Part model, mm, in its own coordinate system. A direction names the side the tool comes from. Give positions to 0.01 mm unless a question says otherwise; leave off trailing zeros. Loops run counter-clockwise (first coordinate to the right, second up) from the corner with the lowest first, then second, coordinate; pieces in that order, holes last. Notation, with made-up numbers: (32.5, 27) -> (61.5, 27) arc R16 ccw to (61.5, 51) -> close; hole circle Ø4 at (-14, 66). An arc over 180 degrees is marked (long way). One line per question, with ' | ' between items.
```python
from build123d import *

# Parameters (mm, degrees)
ESQUISSE1_R                  = 2.5
BOSS_EXTRU_1_DEPTH           = 15
ESQUISSE2_W                  = 3.3
ESQUISSE2_H                  = 15.5
ENL_V_MAT_EXTRU_1_DEPTH      = 3.5
ENL_V_MAT_EXTRU_1_DEPTH_BACK = 12.5
ESQUISSE5_R                  = 2.5
ENL_V_MAT_EXTRU_4_DEPTH      = 10
ESQUISSE6_R                  = 5.5
ESQUISSE6_R_2                = 2.5
BOSS_EXTRU_2_DEPTH           = 3
ENL_V_MAT_EXTRU_5_DEPTH      = 3


with BuildPart() as part:
    # Esquisse1 → Boss.-Extru.1 (new body)
    with BuildSketch(Plane.XY):
        with BuildLine():
            Line((-4.5, -1.302598386), (-4.5, -17))
            Line((-4.5, -17), (-1.6, -17))
            Line((-1.6, -17), (-1.6, -1.302598386))
            Line((-1.6, -1.302598386), (1.6, -1.302598386))
            Line((1.6, -1.302598386), (1.6, -17))
            Line((1.6, -17), (4.5, -17))
            Line((4.5, -17), (4.5, -1.302598386))
            Line((4.5, -1.302598386), (6, -1.302598386))
            Line((6, -1.302598386), (6, 6.394448725))
            ThreePointArc((6, 6.394448725), (0, 3), (-6, 6.394448725))
            Line((-6, 6.394448725), (-6, -1.302598386))
            Line((-6, -1.302598386), (-4.5, -1.302598386))
        make_face()
        with BuildLine():
            Line((-6, 13.605551275), (-6, 6.394448725))
            ThreePointArc((-6, 6.394448725), (0, 3), (6, 6.394448725))
            Line((6, 6.394448725), (6, 13.605551275))
            ThreePointArc((6, 13.605551275), (3.446820352, 16.092571663), (0, 17))
            ThreePointArc((0, 17), (-3.446820352, 16.092571663), (-6, 13.605551275))
        make_face()
        with Locations((0, 10)):
            Circle(ESQUISSE1_R, mode=Mode.SUBTRACT)
        with BuildLine():
            Line((6, 13.605551275), (6, 6.394448725))
            ThreePointArc((6, 6.394448725), (6.745368782, 8.129171307), (7, 10))
            ThreePointArc((7, 10), (6.745368782, 11.870828693), (6, 13.605551275))
        make_face()
        with BuildLine():
            ThreePointArc((-6, 13.605551275), (-7, 10), (-6, 6.394448725))
            Line((-6, 6.394448725), (-6, 13.605551275))
        make_face()
    extrude(amount=BOSS_EXTRU_1_DEPTH)

    # Esquisse2 → Enlèv. mat.-Extru.1 (cut, two sides)
    with BuildSketch(Plane(origin=(4.5, 0, 0), x_dir=(0, 0, -1), z_dir=(1, 0, 0))) as enl_v_mat_extru_1_sk:
        with Locations((-10.5, 9.25)):
            Rectangle(ESQUISSE2_W, ESQUISSE2_H)
        with Locations((-4.5, 9.25)):
            Rectangle(ESQUISSE2_W, ESQUISSE2_H)
    extrude(amount=ENL_V_MAT_EXTRU_1_DEPTH, mode=Mode.SUBTRACT)
    extrude(enl_v_mat_extru_1_sk.sketch, amount=-ENL_V_MAT_EXTRU_1_DEPTH_BACK, mode=Mode.SUBTRACT)

    # Esquisse5 → Enlèv. mat.-Extru.4 (cut)
    with BuildSketch(Plane(origin=(4.5, 0, 0), x_dir=(0, 0, -1), z_dir=(1, 0, 0))):
        with BuildLine():
            ThreePointArc((-7.5, -17), (-12.803300859, -14.803300859), (-15, -9.5))
            Line((-15, -9.5), (-15, -17))
            Line((-15, -17), (-7.5, -17))
        make_face()
        with BuildLine():
            Line((0, -17), (0, -9.5))
            ThreePointArc((0, -9.5), (-2.196699141, -14.803300859), (-7.5, -17))
            Line((-7.5, -17), (0, -17))
        make_face()
        with Locations((-7.5, -9.5)):
            Circle(ESQUISSE5_R)
    extrude(amount=-ENL_V_MAT_EXTRU_4_DEPTH, mode=Mode.SUBTRACT)

    # Esquisse6 → Boss.-Extru.2 (add)
    with BuildSketch(Plane(origin=(0, 0, 0), x_dir=(-1, 0, 0), z_dir=(0, 0, -1))):
        with Locations((0, 10)):
            Circle(ESQUISSE6_R)
        with Locations((0, 10)):
            Circle(ESQUISSE6_R_2, mode=Mode.SUBTRACT)
    extrude(amount=BOSS_EXTRU_2_DEPTH)

    # Esquisse7 → Enlèv. mat.-Extru.5 (cut)
    with BuildSketch(Plane(origin=(0, 0, -3), x_dir=(-1, 0, 0), z_dir=(0, 0, -1))):
        Polygon((0, 14.70707265), (3.897114317, 12.45707265), (3.897114317, 7.95707265), (0, 5.70707265), (-3.897114317, 7.95707265), (-3.897114317, 12.45707265), align=None)
    extrude(amount=-ENL_V_MAT_EXTRU_5_DEPTH, mode=Mode.SUBTRACT)


solid = part.part
```
1) Saw through at B-B (z = 7). Give the cut face in (x, y), and give its area (3 significant figures).
Found:
outline: (-6, -1.3) -> (-4.5, -1.3) -> (-4.5, -7.05) -> (-1.6, -7.05) -> (-1.6, -1.3) -> (1.6, -1.3) -> (1.6, -7.05) -> (4.5, -7.05) -> (4.5, -1.3) -> (6, -1.3) -> (6, 6.39) arc R7 ccw (long way) to (-6, 6.39) -> close; (-4.5, -16.98) -> (-1.6, -16.98) -> (-1.6, -11.95) -> (-4.5, -11.95) -> close; (1.6, -16.98) -> (4.5, -16.98) -> (4.5, -11.95) -> (1.6, -11.95) -> close; hole circle Ø5 at (0, 10) | area: 260 mm2
2) Saw through at C-C (x = 1.25). State how many separate pieces and enclosed holes the cut face has, and give its area (3 significant figures).
Found:
separate pieces: 4 | enclosed holes: 0 | area: 144 mm2
3) Pin check, flat tips, straight feed: P1, Ø8, axis at y = -9.5, z = 7.5, coming from the +X side; P2, Ø3.5, axis at y = 10, z = -2, coming from the +X side; P3, Ø3, axis at x = -2.5, z = 7.5, coming from the +Y side. Stop position of each tip, or through.
Found:
P1: x = 4.5 | P2: x = 5.5 | P3: y = 16.93
4) Saw through at D-D (y = -11). Give the cut face in (x, z).
Found:
outline: (-4.5, 0.15) -> (-1.6, 0.15) -> (-1.6, 5.5) -> (-4.5, 5.5) -> close; (-4.5, 9.5) -> (-1.6, 9.5) -> (-1.6, 14.85) -> (-4.5, 14.85) -> close; (1.6, 0.15) -> (4.5, 0.15) -> (4.5, 5.5) -> (1.6, 5.5) -> close; (1.6, 9.5) -> (4.5, 9.5) -> (4.5, 14.85) -> (1.6, 14.85) -> close
5) Drill centre lines: line 1 (Z direction, x = 2, y = 15); line 2 (Z direction, x = 0, y = 14); line 3 (X direction, y = -7.5, z = 5.75). Where is each one in solid material? Low to high.
Found:
line 1: -3 to 2.85, 6.15 to 8.85, 12.15 to 15 | line 2: 0 to 2.85, 6.15 to 8.85, 12.15 to 15 | line 3: -4.5 to -1.6, 1.6 to 4.5
6) Pull direction Y, two halves, no side cores. Call faces 5 (the flat face through (-5, -1.303, 7)), 6 (the flat face through (1.921, 6.816, -1.521)), 7 (the flat face through (6, 2, 7)): pulls with the +Y half, pulls with the -Y half, needs draft (parallel to the pull), parting line crosses it, or undercut.
Found:
face 5: pulls with the -Y half | face 6: undercut | face 7: needs draft
7) Saw through at A-A (y = -3.5). Give the cut face in (x, z), and give its area (3 significant figures).
Found:
outline: (-4.5, 0) -> (-1.6, 0) -> (-1.6, 15) -> (-4.5, 15) -> close; (1.6, 0) -> (4.5, 0) -> (4.5, 15) -> (1.6, 15) -> close | area: 87.0 mm2
8) Tool access for faces 1 (the flat face through (0, 1.5, 11)), 2 (the flat face through (-1.6, -7.5, 5.7)), 3 (the flat face through (-3, 10, 0)), 4 (the flat face through (4.5, -7.5, 5.7)): list every direction of +Z, -Z, +X, -X, +Y, -Y with a clear straight run to the whole face (end or side of a thin tool).
Found:
face 1: +X, -X, +Y | face 2: +Z, -Z, -Y | face 3: -Z | face 4: +Z, -Z, +X, -Y
